```python
from build123d import *

# Parameters (mm, degrees)
SKETCH1_W           = 9.5
SKETCH1_H           = 30
BOSS_EXTRUDE1_DEPTH = 5
SKETCH2_R           = 3.1
SKETCH2_R_2         = 1.7
CUT_EXTRUDE1_DEPTH  = 17.509466981
BOSS_EXTRUDE3_START = -3.2
SKETCH8_R           = 3.1
BOSS_EXTRUDE3_DEPTH = 3.2
CHAMFER1_SIZE       = 0.5
BOSS_EXTRUDE2_DEPTH = 5
CUT_EXTRUDE2_DEPTH  = 50.658836072
SKETCH6_R           = 1.3
CUT_EXTRUDE3_DEPTH  = 45.788689937
SKETCH9_W           = 2.39154787
SKETCH9_H           = 2.527864045
CUT_EXTRUDE4_DEPTH  = 50.658836072
FILLET2_R           = 1.5
FILLET1_R           = 5
SKETCH10_R          = 3.25
CUT_EXTRUDE5_DEPTH  = 2
SKETCH13_R          = 1.25
CUT_EXTRUDE6_DEPTH  = 49.301239371
FILLET3_R           = 0.5


with BuildPart() as part:
    # Sketch1 → Boss-Extrude1 (new body)
    with BuildSketch(Plane(origin=(0, 0, 0), x_dir=(1, 0, 0), z_dir=(0, 1, 0))):
        Rectangle(SKETCH1_W, SKETCH1_H)
    extrude(amount=BOSS_EXTRUDE1_DEPTH)

    # Sketch2 → Cut-Extrude1 (cut, through all)
    with BuildSketch(Plane(origin=(0, 5, 0), x_dir=(1, 0, 0), z_dir=(0, 1, 0))):
        with Locations(Location((0, 9, 0), (0, 0, 270))):
            Circle(SKETCH2_R)
        with Locations(Location((0, 0, 0), (0, 0, 270))):
            Circle(SKETCH2_R_2)
        with Locations(Location((0, -9, 0), (0, 0, 270))):
            Circle(SKETCH2_R)
    extrude(amount=-CUT_EXTRUDE1_DEPTH, mode=Mode.SUBTRACT)

    # Sketch8 → Boss-Extrude3 (add)
    with BuildSketch(Plane.XZ.offset(BOSS_EXTRUDE3_START)):
        with Locations(Location((0, 9, 0), (0, 0, 90))):
            Circle(SKETCH8_R)
        with Locations(Location((0, -9, 0), (0, 0, 90))):
            Circle(SKETCH8_R)
    extrude(amount=BOSS_EXTRUDE3_DEPTH)

    # Chamfer1
    chamfer1_edges = [part.edges().sort_by_distance(p)[0] for p in [
        (0, 5, -12.1),
        (0, 5, 5.9),
    ]]
    chamfer(chamfer1_edges, length=CHAMFER1_SIZE)

    # Sketch3 → Boss-Extrude2 (add)
    with BuildSketch(Plane(origin=(0, 5, 0), x_dir=(1, 0, 0), z_dir=(0, 1, 0))):
        Polygon((-4.75, 15), (-4.75, 19), (-4.75, 29), (35.25, 29), (35.25, 19), (4.75, 19), (4.75, 15), align=None)
    extrude(amount=-BOSS_EXTRUDE2_DEPTH)

    # Sketch5 → Cut-Extrude2 (cut, through all)
    with BuildSketch(Plane(origin=(35.25, 0, 0), x_dir=(0, 0, -1), z_dir=(1, 0, 0))):
        Polygon((19, 5), (29, 1.750803038), (29, 5), align=None)
    extrude(amount=-CUT_EXTRUDE2_DEPTH, mode=Mode.SUBTRACT)

    # Sketch6 → Cut-Extrude3 (cut, through all)
    with BuildSketch(Plane(origin=(0, 10.106502383, -3.283801684), x_dir=(1, 0, 0), z_dir=(0, 0.9510565162951556, -0.30901699437494123))):
        with Locations(Location((-0.75, 20.524988838, 0), (0, 0, 270))):
            Circle(SKETCH6_R)
        with Locations(Location((31.25, 20.524988838, 0), (0, 0, 270))):
            Circle(SKETCH6_R)
    extrude(amount=-CUT_EXTRUDE3_DEPTH, mode=Mode.SUBTRACT)

    # Sketch9 → Cut-Extrude4 (cut, through all)
    with BuildSketch(Plane(origin=(35.25, 0, 0), x_dir=(0, 0, -1), z_dir=(1, 0, 0))):
        with Locations((27.804226065, 1.263932023)):
            Rectangle(SKETCH9_W, SKETCH9_H)
    extrude(amount=-CUT_EXTRUDE4_DEPTH, mode=Mode.SUBTRACT)

    # Fillet2
    fillet2_edges = [part.edges().sort_by_distance(p)[0] for p in [
        (35.25, 2.5, -19),
        (4.75, 2.5, 15),
        (-4.75, 2.5, 15),
        (35.25, 1.263932023, -26.60845213),
        (-4.75, 1.263932023, -26.60845213),
    ]]
    fillet(fillet2_edges, radius=FILLET2_R)

    # Fillet1
    fillet1_edges = [part.edges().sort_by_distance(p)[0] for p in [
        (4.75, 2.5, -19),
    ]]
    fillet(fillet1_edges, radius=FILLET1_R)

    # Sketch10 → Cut-Extrude5 (cut)
    with BuildSketch(Plane.XZ):
        with Locations(Location((0, 0, 0), (0, 0, 270))):
            Circle(SKETCH10_R)
    extrude(amount=-CUT_EXTRUDE5_DEPTH, mode=Mode.SUBTRACT)

    # Sketch13 → Cut-Extrude6 (cut, through all)
    with BuildSketch(Plane.ZY.offset(4.75)):
        with Locations((-3.55, 5)):
            Circle(SKETCH13_R)
        with Locations((3.55, 5)):
            Circle(SKETCH13_R)
    extrude(amount=-CUT_EXTRUDE6_DEPTH, mode=Mode.SUBTRACT)

    # Fillet3
    fillet3_edges = [part.edges().sort_by_distance(p)[0] for p in [
        (0, 5, -4.8),
        (0, 5, -2.3),
        (0, 5, 4.8),
        (0, 5, 2.3),
    ]]
    fillet(fillet3_edges, radius=FILLET3_R)


solid = part.part
```
Verification items for the finished model (mm, model axes). A direction names the side the tool comes from. Give positions to 0.01 mm unless a question says otherwise; leave off trailing zeros. Order: outer loops, then holes, each group sorted by start corner. A loop starts at its lowest first (then second) coordinate and runs counter-clockwise, first axis right, second up. Notation, with made-up numbers: (-15.5, 26.5) -> (-9.5, 26.5) arc R15 cw to (-9.5, 32.5) -> close; hole circle Ø11 at (20, 5). An arc over 180 degrees is marked (long way). One line per item, written item: value.
(1) Scan lines: line 1 along X through (y, z) = (3.75, -9); line 2 along X through (y, z) = (3.7, 0); line 3 along X through (y, z) = (1.6, 7). Record each from-to range of solid material in increasing order. Write a range as [from, to].
Final values:
line 1: [-4.75, -3.1], [3.1, 4.75]
line 2: [-4.75, -1.7], [1.7, 4.75]
line 3: [-4.75, 4.75]
(2) Tool access check on faces 4 (the face through (0, 3.2, 9)), 5 (the face through (-1.978, 0.986, 2.579)), 6 (the face through (4.75, 3, 0)). Record the directions out of +Z, -Z, +X, -X, +Y, -Y that give a thin tool (end or side, any length) a straight path to the whole face; none if there is none.
Final values:
face 4: +Y
face 5: -Y
face 6: +Z, +X, +Y, -Y
(3) Gauge pin test, flat ends, axial feed: pin 1 (5 mm diameter, centred on x = 0, z = 9, fed in from +Y); pin 2 (1.5 mm diameter, centred on y = 3.5, z = 2.5, fed in from +X); pin 3 (2 mm diameter, centred on x = 22.5, y = 0.5, fed in from +Z). Record the tip position at first contact, or that the pin passes through.
Final values:
pin 1: y = 3.2
pin 2: x = 4.75
pin 3: z = -19
(4) Sectioned sample at C-C on x = 0. Count the separate pieces of the cut face and the enclosed holes in it, then the cut area to 3 significant figures.
Final values:
separate pieces: 3
enclosed holes: 0
area: 139 mm^2
(5) Draft check along Z on faces 1 (the face through (0, 5, 13)), 2 (the face through (4.3, 2.54, 14.57)), 3 (the face through (-0.07, 3.75, -3.57)). Enter one of: pulls with the +Z half, pulls with the -Z half, needs draft (parallel to the pull), parting line crosses it, or undercut.
Final values:
face 1: needs draft
face 2: pulls with the +Z half
face 3: undercut
(6) Sectioned sample at A-A on z = 0. Record the cut outline in (x, y).
Final values:
outline: (-4.75, 0) -> (-3.25, 0) -> (-3.25, 2) -> (-1.7, 2) -> (-1.7, 5) -> (-4.75, 5) -> close; (1.7, 2) -> (3.25, 2) -> (3.25, 0) -> (4.75, 0) -> (4.75, 5) -> (1.7, 5) -> close
(7) Sectioned sample at B-B on z = 9. Record the cut outline in (x, y).
Final values:
outline: (-4.75, 0) -> (4.75, 0) -> (4.75, 5) -> (3.6, 5) -> (3.1, 4.5) -> (3.1, 3.2) -> (-3.1, 3.2) -> (-3.1, 4.5) -> (-3.6, 5) -> (-4.75, 5) -> close
